Geometry: final body of the model. Coordinates: model frame, mm. Coordinates: 2 decimals unless noted, no trailing zeros. Write each loop counter-clockwise with the first axis right and the second up, starting at its lowest first coordinate (ties: lowest second). Pieces come first, ordered by that corner, then holes. Notation, with made-up numbers: M -30,56 L -5,56 A24 ccw -5,82 Z; hole C -3.5,-27.75 d3. An arc over 180 degrees is marked long. Write item = value, one per line. Start each with the question number.
Item 1: Pull-direction query (Y, two-part tool) for faces 1 (the cylindrical face through (-36, 65.9, 116.9)), 2 (the cylindrical face through (-36, 61.41, 61.34)), 3 (the cylindrical face through (-35.93, 139.65, 137.75)), 4 (the cylindrical face through (-35.91, -68.66, 50.37)); classes: +Y half, -Y half, draft (parallel to the pull), parting line (faces both ways), or undercut.
Item 2: Section B-B on z = 100. Output: boundary loops of the cut face in (x, y), plus the area to 3 significant figures.
Item 3: Section C-C on x = -36.5. Give the number of separate pieces and of enclosed holes in the cut face, plus the area to 3 significant figures.
Item 4: Section D-D on z = 157. Output: boundary loops of the cut face in (x, y), plus the area to 3 significant figures.
Item 5: First-contact query: pin 1 Ø4 at (y, z) = (59.3, 60) entering from -X; pin 2 Ø1 at (x, y) = (-34.5, 101.5) entering from -Z; pin 3 Ø8 at (y, z) = (45.7, 150) entering from +X. Flat tips, straight axial feed; report the tip coordinate or a pass-through.
Item 6: Ray query, L1, parallel to Y at x = -33.7, z = 85.5; L2, parallel to Y at x = -36.2, z = 150; L3, parallel to Z at x = -38, y = 88.5. Return the intervals inside material, ascending. Write a range as [from, to].
Item 7: Section A-A on z = 123.57. Output: boundary loops of the cut face in (x, y).
from build123d import *

# Parameters (mm, degrees)
SALIENTE_EXTRUIR1_DEPTH = 200
CROQUIS2_R              = 2.5
CORTAR_EXTRUIR1_DEPTH   = 100
CROQUIS3_W              = 4.95
CROQUIS3_H              = 200
SALIENTE_EXTRUIR2_DEPTH = 60
CROQUIS4_R              = 2.5
CROQUIS4_R_2            = 5
CORTAR_EXTRUIR2_DEPTH   = 60
REDONDEO1_R             = 10


with BuildPart() as part:
    # Croquis1 → Saliente-Extruir1 (new body)
    with BuildSketch(Plane.XY):
        Polygon((-38.444023, 46.698845), (-38.444023, -35.401155), (-38.444023, -69.401155), (-33.444023, -69.401155), (-33.444023, -35.401155), (-33.494023, 46.698845), (-33.494023, 80.698845), (-38.444023, 80.698845), align=None)
    extrude(amount=SALIENTE_EXTRUIR1_DEPTH)

    # Croquis2 → Cortar-Extruir1 (cut)
    with BuildSketch(Plane.ZY.offset(38.444023)):
        with Locations((85.5, 65.198845)):
            Circle(CROQUIS2_R)
        with Locations((114.5, 65.198845)):
            Circle(CROQUIS2_R)
        with Locations((50, 45.698845)):
            Circle(CROQUIS2_R)
        with Locations((150, 45.698845)):
            Circle(CROQUIS2_R)
        with Locations((150, -34.401155)):
            Circle(CROQUIS2_R)
        with Locations((114.5, -53.901155)):
            Circle(CROQUIS2_R)
        with Locations((85.5, -53.901155)):
            Circle(CROQUIS2_R)
        with Locations((50, -34.401155)):
            Circle(CROQUIS2_R)
    extrude(amount=-CORTAR_EXTRUIR1_DEPTH, mode=Mode.SUBTRACT)

    # Croquis3 → Saliente-Extruir2 (add)
    with BuildSketch(Plane(origin=(0, 80.698845, 0), x_dir=(1, 0, 0), z_dir=(0, 1, 0))):
        with Locations((-35.969023, -100)):
            Rectangle(CROQUIS3_W, CROQUIS3_H)
    extrude(amount=SALIENTE_EXTRUIR2_DEPTH)

    # Croquis4 → Cortar-Extruir2 (cut)
    with BuildSketch(Plane.ZY.offset(38.444023)):
        with Locations((76.43, 136.068845)):
            Circle(CROQUIS4_R)
        with Locations((123.57, 136.068845)):
            Circle(CROQUIS4_R)
        with Locations((76.43, 88.928845)):
            Circle(CROQUIS4_R)
        with Locations((123.57, 88.928845)):
            Circle(CROQUIS4_R)
        with Locations((100, 112.498845)):
            Circle(CROQUIS4_R_2)
        with Locations((60, 59.298845)):
            Circle(CROQUIS4_R)
        with Locations((140, 59.298845)):
            Circle(CROQUIS4_R)
        Polygon((61.8, 140.698845), (0, 60.698845), (0, 140.698845), align=None)
        Polygon((0, -19.301155), (50, -69.401155), (0, -69.401155), align=None)
        Polygon((200, -19.301155), (150, -69.401155), (200, -69.401155), align=None)
        Polygon((138.2, 140.698845), (200, 60.698845), (200, 140.698845), align=None)
    extrude(amount=-CORTAR_EXTRUIR2_DEPTH, mode=Mode.SUBTRACT)

    # Redondeo1
    redondeo1_edges = [part.edges().sort_by_distance(p)[0] for p in [
        (-35.969023, 60.698845, 0),
        (-35.944023, -69.401155, 50),
        (-35.944023, -69.401155, 150),
        (-35.969023, 60.698845, 200),
        (-35.969023, 140.698845, 138.2),
        (-35.969023, 140.698845, 61.8),
        (-35.948925, -19.301155, 0),
        (-35.948925, -19.301155, 200),
    ]]
    fillet(redondeo1_edges, radius=REDONDEO1_R)


solid = part.part
Responses:
q1.face_1 = undercut
q1.face_2 = undercut
q1.face_3 = +Y half
q1.face_4 = -Y half
q2.outline = M -38.44,-69.4 L -33.44,-69.4 L -33.44,-35.4 L -33.49,46.7 L -33.49,107.5 L -38.44,107.5 Z; M -38.44,117.5 L -33.49,117.5 L -33.49,140.7 L -38.44,140.7 Z
q2.area = 994 mm²
q3.separate_pieces = 1
q3.enclosed_holes = 15
q3.area = 34,200 mm²
q4.outline = M -38.44,-62.39 L -33.44,-62.39 L -33.44,-35.4 L -33.49,46.7 L -33.49,116.36 L -38.44,116.36 Z
q4.area = 888 mm²
q5.pin_1 = through
q5.pin_2 = 31.13
q5.pin_3 = -33.49
q6.L1 = [-69.4, -56.4], [-51.4, 62.7], [67.7, 140.7]
q6.L2 = [-68.5, -36.9], [-31.9, 43.2], [48.2, 125.42]
q6.L3 = [21.48, 73.97], [78.89, 121.11], [126.03, 178.52]
q7.outline = M -38.44,-69.4 L -33.44,-69.4 L -33.44,-35.4 L -33.49,46.7 L -33.49,86.43 L -38.44,86.43 Z; M -38.44,91.43 L -33.49,91.43 L -33.49,133.57 L -38.44,133.57 Z; M -38.44,138.57 L -33.49,138.57 L -33.49,140.7 L -38.44,140.7 Z
